```python
from build123d import *

# Parameters (mm, degrees)
BOSS_EXTRUDE1_DEPTH = 3
SKETCH2_R           = 1.6
CUT_EXTRUDE1_DEPTH  = 3
SKETCH3_W           = 2.188746234
SKETCH3_H           = 3
BOSS_EXTRUDE2_DEPTH = 12.5
SKETCH4_R           = 1.0926154
CUT_EXTRUDE2_DEPTH  = 12.5
SKETCH5_W           = 12.5
SKETCH5_H           = 3
SKETCH5_R           = 1.0926154
BOSS_EXTRUDE3_DEPTH = 2.188746233
SKETCH6_W           = 28.2
SKETCH6_H           = 3
BOSS_EXTRUDE4_DEPTH = 8.9


with BuildPart() as part:
    # Sketch1 → Boss-Extrude1 (new body)
    with BuildSketch(Plane.XY):
        with BuildLine():
            Line((9.576829353, 12.891428571), (37.776829353, 12.891428571))
            Line((37.776829353, 12.891428571), (37.776829353, 29.952191633))
            ThreePointArc((37.776829353, 29.952191633), (36.21300306, 33.727602279), (32.437592415, 35.291428571))
            Line((32.437592415, 35.291428571), (14.916066291, 35.291428571))
            ThreePointArc((14.916066291, 35.291428571), (11.140655646, 33.727602279), (9.576829353, 29.952191633))
            Line((9.576829353, 29.952191633), (9.576829353, 12.891428571))
        make_face()
        with BuildLine():
            Line((14.079239539, 21.646631976), (21.938160435, 16.057593806))
            ThreePointArc((21.938160435, 16.057593806), (23.676829353, 15.502390402), (25.415498271, 16.057593806))
            Line((25.415498271, 16.057593806), (33.274419167, 21.646631976))
            ThreePointArc((33.274419167, 21.646631976), (34.53575025, 24.091428571), (33.274419167, 26.536225167))
            Line((33.274419167, 26.536225167), (25.415498271, 32.125263337))
            ThreePointArc((25.415498271, 32.125263337), (23.676829353, 32.680466741), (21.938160435, 32.125263337))
            Line((21.938160435, 32.125263337), (14.079239539, 26.536225167))
            ThreePointArc((14.079239539, 26.536225167), (12.817908456, 24.091428571), (14.079239539, 21.646631976))
        make_face(mode=Mode.SUBTRACT)
    extrude(amount=BOSS_EXTRUDE1_DEPTH)

    # Sketch2 → Cut-Extrude1 (cut)
    with BuildSketch(Plane.XY.offset(3)):
        with Locations((13.176829353, 30.793016236)):
            Circle(SKETCH2_R)
        with Locations((34.176829353, 30.793016236)):
            Circle(SKETCH2_R)
        with Locations((13.176829353, 16.793016236)):
            Circle(SKETCH2_R)
        with Locations((34.176829353, 16.793016236)):
            Circle(SKETCH2_R)
    extrude(amount=-CUT_EXTRUDE1_DEPTH, mode=Mode.SUBTRACT)

    # Sketch3 → Boss-Extrude2 (add)
    with BuildSketch(Plane(origin=(0, 0, 0), x_dir=(-1, 0, 0), z_dir=(0, 0, -1))):
        with Locations((-23.676829353, 33.791428571)):
            Rectangle(SKETCH3_W, SKETCH3_H)
    extrude(amount=BOSS_EXTRUDE2_DEPTH)

    # Sketch4 → Cut-Extrude2 (cut)
    with BuildSketch(Plane(origin=(24.77120247, 0, 0), x_dir=(0, 0, -1), z_dir=(1, 0, 0))):
        with Locations((6.25, 33.791428571)):
            Circle(SKETCH4_R)
    extrude(amount=-CUT_EXTRUDE2_DEPTH, mode=Mode.SUBTRACT)



with BuildPart() as body_2:
    # Sketch5 → Boss-Extrude3 (new body)
    with BuildSketch(Plane(origin=(24.77120247, 0, 0), x_dir=(0, 0, -1), z_dir=(1, 0, 0))):
        with Locations((6.25, 5.491428571)):
            Rectangle(SKETCH5_W, SKETCH5_H)
        with Locations((6.25, 5.491428571)):
            Circle(SKETCH5_R, mode=Mode.SUBTRACT)
    extrude(amount=-BOSS_EXTRUDE3_DEPTH)


with BuildPart() as part_1:
    add(part.part)

    add(body_2.part)  # Boss-Extrude4 merges body 2
    # Sketch6 → Boss-Extrude4 (add)
    with BuildSketch(Plane.XZ.offset(-12.891428571)):
        with Locations((23.676829353, 1.5)):
            Rectangle(SKETCH6_W, SKETCH6_H)
    extrude(amount=BOSS_EXTRUDE4_DEPTH)


solid = part_1.part
```
Input: part model. Units: mm. Frame: model coordinates. A direction names the side the tool comes from. Round coordinates to 2 decimals unless told otherwise and drop trailing zeros. Loops run counter-clockwise (first coordinate to the right, second up) from the corner with the lowest first, then second, coordinate; pieces in that order, holes last. Notation, with made-up numbers: (18.5, 36.25) - (40.5, 36.25) arc R12 ccw to (40.5, 59.25) - close; hole circle Ø5 at (82.25, -27). An arc over 180 degrees is marked (long way). One line per item, written item: value. Start each with the question number.
(1) Section A-A, the plane z = -2.5. Return loops of the section in (x, y).
(2) Access query for faces 5 (the flat face through (22.582, 35.1, -6.2)), 6 (the cylindrical face through (12.82, 24.13, 1.48)), 7 (the flat face through (24, 6.991, -6)). Directions: +Z, -Z, +X, -X, +Y, -Y. A direction counts if a zero-diameter tool reaches every point of the face in a straight line with its end or side. Return the directions, or none.
(3) Ray query, line 1 (Y direction, x = 23.7, z = -6.25); line 2 (Y direction, x = 24, z = -7); line 3 (Z direction, x = 25.5, y = 34). Return the intervals inside material, ascending. Write a range as [from, to].
(4) Section B-B, the plane y = 24. Return loops of the section in (x, z).
(5) Draft query along X for faces 1 (the cylindrical face through (23.692, 32.725, -6.013)), 2 (the flat face through (17.954, 18.891, 1.479)), 3 (the flat face through (37.777, 17, 1)), 4 (the flat face through (29.4, 29.29, 1.48)). Return one class per face: +X half, -X half, draft (parallel to the pull), parting line (faces both ways), or undercut.
(6) Contact query for flat-ended pins moving along their axis: P1, Ø1.5, axis at y = 5.5, z = -7.5, coming from the -X side; P2, Ø3.5, axis at x = 13.18, y = 30.79, coming from the -Z side; P3, Ø2.5, axis at y = 6, z = -8.5, coming from the +X side. Output: stop coordinate, or through.
(7) Section C-C, the plane z = -6.25. Return loops of the section in (x, y).
(8) Section D-D, the plane y = 31.5. Return loops of the section in (x, z).
Results below:
1. outline: (22.58, 3.99) - (24.77, 3.99) - (24.77, 6.99) - (22.58, 6.99) - close; (22.58, 32.29) - (24.77, 32.29) - (24.77, 35.29) - (22.58, 35.29) - close
2. face 5: -Z, -X, +Y, -Y
2. face 6: +Z, -Z
2. face 7: -Z, +X, -X
3. line 1: [3.99, 4.4], [6.58, 6.99], [32.29, 32.7], [34.88, 35.29]
3. line 2: [3.99, 4.7], [6.29, 6.99], [32.29, 33], [34.59, 35.29]
3. line 3: [0, 3]
4. outline: (9.58, 0) - (12.82, 0) - (12.82, 3) - (9.58, 3) - close; (34.53, 0) - (37.78, 0) - (37.78, 3) - (34.53, 3) - close
5. face 1: draft
5. face 2: undercut
5. face 3: +X half
5. face 4: undercut
6. P1: x = 22.58
6. P2: z = 0
6. P3: x = 24.77
7. outline: (22.58, 3.99) - (24.77, 3.99) - (24.77, 4.4) - (22.58, 4.4) - close; (22.58, 6.58) - (24.77, 6.58) - (24.77, 6.99) - (22.58, 6.99) - close; (22.58, 32.29) - (24.77, 32.29) - (24.77, 32.7) - (22.58, 32.7) - close; (22.58, 34.88) - (24.77, 34.88) - (24.77, 35.29) - (22.58, 35.29) - close
8. outline: (9.81, 0) - (11.74, 0) - (11.74, 3) - (9.81, 3) - close; (14.61, 0) - (21.06, 0) - (21.06, 3) - (14.61, 3) - close; (26.29, 0) - (32.74, 0) - (32.74, 3) - (26.29, 3) - close; (35.61, 0) - (37.55, 0) - (37.55, 3) - (35.61, 3) - close
